Autodesk Inventor part; units mm, degrees
ref_plane "YZ Plane" through (0, 0, 0) normal (1, 0, 0) x (0, 1, 0)
ref_plane "XZ Plane" through (0, 0, 0) normal (0, 1, 0) x (-1, 0, 0)
ref_plane "XY Plane" through (0, 0, 0) normal (0, 0, 1) x (1, 0, 0)
sketch "Sketch1" plane through (0, 0, 0) normal (1, 0, 0) x (0, 1, 0)
  circle A0 centre (0, 0) radius 11.1125
  dimension "d0" = 22.225
extrude "Extrusion1" add sketch "Sketch1" along normal blind 2.54
sketch "Sketch2" plane through (2.54, 0, 0) normal (1, 0, 0) x (0, 0, -1)
  line L0 (-1.524, 1.524) -> (1.524, 1.524)
  line L1 (1.524, 1.524) -> (1.524, -1.524)
  line L2 (1.524, -1.524) -> (-1.524, -1.524)
  line L3 (-1.524, -1.524) -> (-1.524, 1.524)
  point P0 (0, 0)
  dimension "d3" = 3.048
  dimension "d4" = 3.048
  dimension "d5" = 1.524
  dimension "d6" = 1.524
extrude "Extrusion2" add sketch "Sketch2" along normal blind 19.05
sketch "Sketch3" plane through (0, 0, 0) normal (-1, 0, 0) x (0, 0, 1)
  point P0 (0, 0)
  point P1 (-8.001, 0)
  point P2 (8.001, 0)
  dimension "d9" = 16.002
  dimension "d10" = 8.001
hole "Hole1" at (0, 0, 8.001) at (0, 0, -8.001) direction (1, 0, 0) diameter 2.4892 depth 2.54
equation "\"d4\" = d3"
properties part number "vex servo addapter" material "Aluminum 6061"
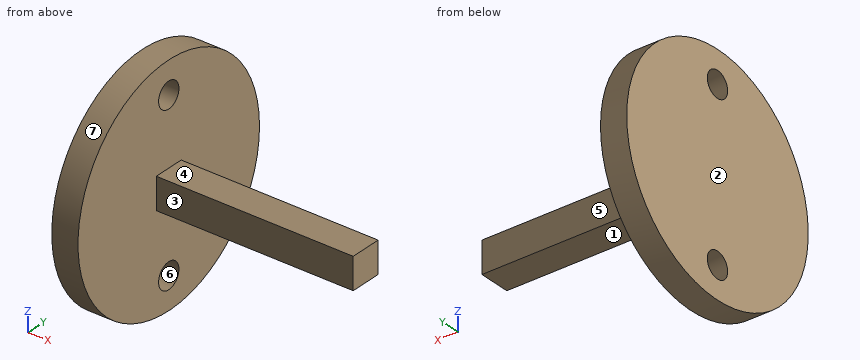
Here's how the part is built. I have some questions about the finished solid (model axes, mm). Face numbers are marked on the shaded views. A direction names the side the tool comes from. Give positions to 0.01 mm unless a question says otherwise; leave off trailing zeros. Write each loop counter-clockwise with the first axis right and the second up, starting at its lowest first coordinate (ties: lowest second). Pieces come first, ordered by that corner, then holes.
(1) Imagine slicing it at A-A, the plane z = 8.25. Write out the boundary of the cut face in (x, y).
Output values:
outline: (0, -7.44) - (2.54, -7.44) - (2.54, -1.22) - (0, -1.22) - close; (0, 1.22) - (2.54, 1.22) - (2.54, 7.44) - (0, 7.44) - close
(2) Imagine slicing it at B-B, the plane y = 0.5. Write out the boundary of the cut face in (x, z), and give its area (3 significant figures).
Output values:
outline: (0, -11.1) - (2.54, -11.1) - (2.54, -9.14) - (0, -9.14) - close; (0, -6.86) - (2.54, -6.86) - (2.54, -1.52) - (21.59, -1.52) - (21.59, 1.52) - (2.54, 1.52) - (2.54, 6.86) - (0, 6.86) - close; (0, 9.14) - (2.54, 9.14) - (2.54, 11.1) - (0, 11.1) - close
area: 103 mm2
(3) Thinking about a two-plate mould opening in Z: for the marked faces 4, 5, 6 and 7, which applies, pulls with the +Z half, pulls with the -Z half, needs draft (parallel to the pull), parting line crosses it, or undercut?
Output values:
face 4: pulls with the +Z half
face 5: needs draft
face 6: undercut
face 7: parting line crosses it
(4) Imagine slicing it at D-D, the plane x = 8. Write out the boundary of the cut face in (y, z).
Output values:
outline: (-1.52, -1.52) - (1.52, -1.52) - (1.52, 1.52) - (-1.52, 1.52) - close
(5) On a 3-axis mill with a long thin cutter (end or side, diameter ignored), from which of +Z, -Z, +X, -X, +Y, -Y can I reach the whole of each face in a straight line? I mean the marked faces 1, 2 and 3. Say none if no direction works.
Output values:
face 1: -Z, +X, +Y, -Y
face 2: +Z, -Z, -X, +Y, -Y
face 3: +Z, -Z, +X, -Y
(6) Imagine slicing it at C-C, the plane z = 0. Write out the boundary of the cut face in (x, y).
Output values:
outline: (0, -11.11) - (2.54, -11.11) - (2.54, -1.52) - (21.59, -1.52) - (21.59, 1.52) - (2.54, 1.52) - (2.54, 11.11) - (0, 11.11) - close
(7) Will these pins go through, and if not, where does the flat tip stop? pin 1 (1.5 mm diameter, centred on x = 12.5, z = -0.5, fed in from +Y); pin 2 (4 mm diameter, centred on x = 4, y = 8.5, fed in from +Z); pin 3 (0.9 mm diameter, centred on x = 14.5, z = 0, fed in from -Y).
Output values:
pin 1: stops at y = 1.52
pin 2: stops at z = 8.52
pin 3: stops at y = -1.52
(8) If I drill on L1, parallel to Z at x = 1.35, y = 0; L2, parallel to Y at x = 3, z = -0.25; L3, parallel to X at y = 4.5, z = -2.25, over which ranges is the centre line in solid material (lowest first)?
Output values:
L1: z = -11.11 to -9.25, -6.76 to 6.76, 9.25 to 11.11
L2: y = -1.52 to 1.52
L3: x = 0 to 2.54
